```python
from build123d import *

# Parameters (mm, degrees)
SKETCH1_W               = 66
SKETCH1_H               = 66
BOSS_EXTRUDE1_DEPTH     = 5
SKETCH2_W               = 66
SKETCH2_H               = 66
SKETCH2_W_2             = 60.3
SKETCH2_H_2             = 60.3
BOSS_EXTRUDE2_DEPTH     = 10
CUT_EXTRUDE1_DEPTH      = 55.203320931
CUT_EXTRUDE1_DEPTH_BACK = 55.203320931
SKETCH3_W               = 60.3
SKETCH3_H               = 15
BOSS_EXTRUDE3_REACH     = 100.249
BOSS_EXTRUDE3_START     = -40
SKETCH5_W               = 2.85
SKETCH5_H               = 57.275649276
BOSS_EXTRUDE4_START     = -40
BOSS_EXTRUDE4_DEPTH     = 27.272078
CUT_EXTRUDE2_DEPTH      = 88.796868052
CUT_EXTRUDE2_DEPTH_BACK = 88.796868052
CUT_EXTRUDE3_DEPTH      = 85.308955633
CUT_EXTRUDE3_DEPTH_BACK = 85.308955633
SKETCH12_R              = 2.25


with BuildPart() as part:
    # Sketch1 → Boss-Extrude1 (new body)
    with BuildSketch(Plane(origin=(0, 0, 0), x_dir=(1, 0, 0), z_dir=(0, 0.7071067811865475, 0.7071067811865477))):
        Rectangle(SKETCH1_W, SKETCH1_H)
    extrude(amount=BOSS_EXTRUDE1_DEPTH)

    # Sketch2 → Boss-Extrude2 (add)
    with BuildSketch(Plane(origin=(0, 3.535533906, 3.535533906), x_dir=(1, 0, 0), z_dir=(0, 0.7071067811865476, 0.7071067811865476))):
        Rectangle(SKETCH2_W, SKETCH2_H)
        Rectangle(SKETCH2_W_2, SKETCH2_H_2, mode=Mode.SUBTRACT)
    extrude(amount=BOSS_EXTRUDE2_DEPTH)

    # Sketch3 → Cut-Extrude1 (cut, two sides: drawn at the far end of the back side and taken through both)
    with BuildSketch(Plane(origin=(0, 3.535533906, 3.535533906), x_dir=(1, 0, 0), z_dir=(0, 0.7071067811865476, 0.7071067811865476)).offset(-CUT_EXTRUDE1_DEPTH_BACK)):
        with Locations((0, -22.65)):
            Rectangle(SKETCH3_W, SKETCH3_H)
        with Locations((0, 22.65)):
            Rectangle(SKETCH3_W, SKETCH3_H)
    extrude(amount=CUT_EXTRUDE1_DEPTH + CUT_EXTRUDE1_DEPTH_BACK, mode=Mode.SUBTRACT)

    # Boss-Extrude3: up to this plane
    boss_extrude3_end = Plane(origin=(0, 0, 0), z_dir=(0, -0.7071067811865475, -0.7071067811865477))
    # Sketch5 → Boss-Extrude3 (add, up to the surface)
    with BuildSketch(Plane.XY.offset(BOSS_EXTRUDE3_START), mode=Mode.PRIVATE) as boss_extrude3_sk1:
        with Locations((-31.575, 5.303300859)):
            Rectangle(SKETCH5_W, SKETCH5_H)
    boss_extrude3_tool1 = split(extrude(boss_extrude3_sk1.sketch, amount=BOSS_EXTRUDE3_REACH, mode=Mode.PRIVATE), bisect_by=boss_extrude3_end, keep=Keep.BOTH, mode=Mode.PRIVATE)
    add(boss_extrude3_tool1.solids().sort_by_distance((-31.575, 5.303301, -40))[0])
    # Sketch5 → Boss-Extrude3 (add, up to the surface)
    with BuildSketch(Plane.XY.offset(BOSS_EXTRUDE3_START), mode=Mode.PRIVATE) as boss_extrude3_sk2:
        with Locations((31.575, 5.303300859)):
            Rectangle(SKETCH5_W, SKETCH5_H)
    boss_extrude3_tool2 = split(extrude(boss_extrude3_sk2.sketch, amount=BOSS_EXTRUDE3_REACH, mode=Mode.PRIVATE), bisect_by=boss_extrude3_end, keep=Keep.BOTH, mode=Mode.PRIVATE)
    add(boss_extrude3_tool2.solids().sort_by_distance((31.575, 5.303301, -40))[0])

    # Sketch8 → Boss-Extrude4 (add)
    with BuildSketch(Plane.XY.offset(BOSS_EXTRUDE4_START)):
        Polygon((-33, 33.941125497), (-33, 23.334523779), (-30.15, 23.334523779), (-30.15, 30.941125497), (30.15, 30.941125497), (30.15, 23.334523779), (33, 23.334523779), (33, 33.941125497), (30.15, 33.941125497), (-30.15, 33.941125497), align=None)
    extrude(amount=BOSS_EXTRUDE4_DEPTH)

    # Sketch9 → Cut-Extrude2 (cut, two sides: drawn at the far end of the back side and taken through both)
    with BuildSketch(Plane(origin=(0, 0, -40), x_dir=(-1, 0, 0), z_dir=(0, 0, -1)).offset(-CUT_EXTRUDE2_DEPTH_BACK)):
        Polygon((30.15, 23.334523779), (30.15, 30.941125497), (-30.15, 30.941125497), (-30.15, 23.334523779), (-30.15, 21.319269453), (30.15, 21.319269453), align=None)
    extrude(amount=CUT_EXTRUDE2_DEPTH + CUT_EXTRUDE2_DEPTH_BACK, mode=Mode.SUBTRACT)

    # Sketch12 → Cut-Extrude3 (cut, two sides: drawn at the far end of the back side and taken through both)
    with BuildSketch(Plane.ZY.offset(33).offset(-CUT_EXTRUDE3_DEPTH_BACK)):
        with Locations((-30, 23.941125497)):
            Circle(SKETCH12_R)
        with Locations((-30, -12.058874503)):
            Circle(SKETCH12_R)
        with Locations((-30, 11.941125497)):
            Circle(SKETCH12_R)
        with Locations((-30, -0.058874503)):
            Circle(SKETCH12_R)
    extrude(amount=CUT_EXTRUDE3_DEPTH + CUT_EXTRUDE3_DEPTH_BACK, mode=Mode.SUBTRACT)


solid = part.part
```
Work out the finished part from the listing and answer in its coordinate system (mm). A direction names the side the tool comes from. Coordinates: 2 decimals unless noted, no trailing zeros. Write each loop counter-clockwise with the first axis right and the second up, starting at its lowest first coordinate (ties: lowest second). Pieces come first, ordered by that corner, then holes.
Q1. Find the intervals of material crossed by line 1 (Y direction, x = 31.1, z = -30); line 2 (X direction, y = -17, z = 20.5), in increasing order.
Q2. A cutting plane is placed at B-B, the plane y = 15.5. Give the vertices of the cut face in (x, z), then the cut area to 3 significant figures.
Q3. Which of the six approach directions +Z, -Z, +X, -X, +Y, -Y give full straight-line access (tool end or side, diameter ignored) to faces 1 (the face through (-0.42, -16.09, 26.55)), 2 (the face through (-31.555, 0.617, -27.854)), 3 (the face through (0, 0, 0))?
Q4. Each of these flat-tipped pins is pushed along its axis until it touches: pin 1 Ø8.5 at (x, z) = (0.5, -22.5) entering from -Y; pin 2 Ø4 at (x, y) = (-3.5, -11.5) entering from -Z; pin 3 Ø1.5 at (x, z) = (18.5, -4.5) entering from +Y; pin 4 Ø4 at (y, z) = (-12.06, -30) entering from +X. Where does it stop, or does it pass through?
Q5. Determine the mould class of faces 4 (the face through (31.595, 9.945, -28.962)), 5 (the face through (-30.15, -2, -13)), 6 (the face through (-0.422, 3.686, 3.386)) for opening direction Y: released by +Y, released by -Y, zero draft, split by the parting line, or undercut.
Q6. A cutting plane is placed at C-C, the plane z = -30. State how many separate pieces and enclosed holes the cut face has, then the cut area to 3 significant figures.
Q7. A cutting plane is placed at D-D, the plane y = 8. Give the vertices of the cut face in (x, z), then the cut area to 3 significant figures.
Q8. A cutting plane is placed at A-A, the plane x = -7. Give the vertices of the cut face in (y, z), then the cut area to 3 significant figures.
Findings below:
1. line 1: y = -23.33 to -14.31, -9.81 to -2.31, 2.19 to 9.69, 14.19 to 21.69, 26.19 to 33.94
1. line 2: x = -33 to -30.15, 30.15 to 33
2. outline: (-33, -40) - (-30.15, -40) - (-30.15, 5.71) - (-33, 5.71) - close; (30.15, -40) - (33, -40) - (33, 5.71) - (30.15, 5.71) - close
2. area: 261 mm2
3. face 1: -Z, +Y
3. face 2: +X, -X
3. face 3: -Z, -Y
4. pin 1: stops at y = 30.94
4. pin 2: stops at z = 9.5
4. pin 3: stops at y = 12.32
4. pin 4: passes through
5. face 4: undercut
5. face 5: zero draft
5. face 6: released by +Y
6. separate pieces: 9
6. enclosed holes: 0
6. area: 405 mm2
7. outline: (-33, -40) - (-30.15, -40) - (-30.15, -8) - (30.15, -8) - (30.15, -40) - (33, -40) - (33, 13.21) - (30.15, 13.21) - (30.15, -0.93) - (-30.15, -0.93) - (-30.15, 13.21) - (-33, 13.21) - close
7. area: 730 mm2
8. outline: (-23.33, 23.33) - (-21.32, 21.32) - (-10.71, 31.93) - (-12.73, 33.94) - close; (-10.71, 10.71) - (10.71, -10.71) - (14.25, -7.18) - (-7.18, 14.25) - close; (30.94, -40) - (33.94, -40) - (33.94, -12.73) - (31.93, -10.71) - (30.94, -11.7) - close
8. area: 280 mm2
